Design review of the part built by this model. Coordinates are the model's own, in mm. Face numbers are marked on the shaded views. A direction names the side the tool comes from. Round coordinates to 2 decimals unless told otherwise and drop trailing zeros. Loops run counter-clockwise (first coordinate to the right, second up) from the corner with the lowest first, then second, coordinate; pieces in that order, holes last. Notation, with made-up numbers: M 9,-7 L 19,-7 A33 ccw 19,24 Z; hole C 17.5,87 d9. An arc over 180 degrees is marked long. Use a Markdown table: item, result.
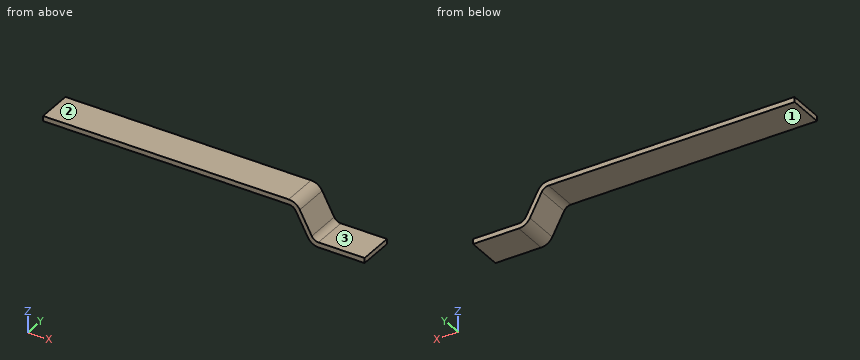
from build123d import *

# Parameters (mm, degrees)
F0_W     = 2
F0_H     = 0.2
F1_DEPTH = 1.4
F2_R     = 0.3
F3_R     = 0.5


with BuildPart() as f1:
    # F0 (on Front) → F1 (new body)
    with BuildSketch(Plane.XZ):
        Polygon((5, 0.1), (-5, 0.1), (-5, -0.1), (4.898743, -0.1), (5, -0.1), align=None)
        Polygon((5.7, -1.2), (5, 0.1), (5, -0.1), (4.898743, -0.1), (5.592507, -1.399263), (5.7, -1.4), align=None)
        with Locations((6.7, -1.3)):
            Rectangle(F0_W, F0_H)
    extrude(amount=F1_DEPTH)

    # F2
    f2_edges = [f1.edges().sort_by_distance(p)[0] for p in [
        (5.7, -0.7, -1.2),
        (4.898743, -0.7, -0.1),
    ]]
    fillet(f2_edges, radius=F2_R)

    # F3
    f3_edges = [f1.edges().sort_by_distance(p)[0] for p in [
        (5, -0.7, 0.1),
        (5.592507, -0.7, -1.399263),
    ]]
    fillet(f3_edges, radius=F3_R)


solid = f1.part
1. Take a section at B-B on z = -0.4. Give the boundary of the cut face in (x, y), and give its area (3 significant figures).
Check values:
| item | result |
|---|---|
| outline | M 5.06,-1.4 L 5.27,-1.4 L 5.27,0 L 5.06,0 Z |
| area | 0.294 mm² |
2. Take a section at A-A on x = -4. Give the boundary of the cut face in (y, z).
Check values:
| item | result |
|---|---|
| outline | M -1.4,-0.1 L 0,-0.1 L 0,0.1 L -1.4,0.1 Z |
3. Machinability: for the marked faces 1, 2 and 3, which of the approach directions +Z, -Z, +X, -X, +Y, -Y give a long, thin tool a straight path to every point of the face, cutting with its end or side? Answer none if there is none.
Check values:
| item | result |
|---|---|
| face 1 | -Z, -X, +Y, -Y |
| face 2 | +Z, +X, -X, +Y, -Y |
| face 3 | +Z, +X, +Y, -Y |
4. Wall thickness on line 1 along Z through (x, y) = (-0.5, -0.55); line 2 along Z through (x, y) = (6.5, -1); line 3 along X through (y, z) = (-0.7, -0.25): over which ranges is each line inside the solid? List them lowest first. Write a range as from..to.
Check values:
| item | result |
|---|---|
| line 1 | z = -0.1..0.1 |
| line 2 | z = -1.4..-1.2 |
| line 3 | x = 4.98..5.19 |
